```python
from build123d import *

# Parameters (mm, degrees)
SKETCH1_W           = 11.8
SKETCH1_H           = 11.8
BOSS_EXTRUDE1_DEPTH = 10
SKETCH2_R           = 10
BOSS_EXTRUDE2_DEPTH = 3
SKETCH3_R           = 4
BOSS_EXTRUDE3_DEPTH = 15
FILLET1_R           = 0.5
FILLET2_R           = 1.5
CUT_EXTRUDE1_REACH  = 44.389
SKETCH6_R           = 1.1


with BuildPart() as part:
    # Sketch1 → Boss-Extrude1 (new body)
    with BuildSketch(Plane(origin=(0, 0, 0), x_dir=(1, 0, 0), z_dir=(0, 1, 0))):
        Rectangle(SKETCH1_W, SKETCH1_H)
    extrude(amount=BOSS_EXTRUDE1_DEPTH)

    # Sketch2 → Boss-Extrude2 (add)
    with BuildSketch(Plane(origin=(0, 10, 0), x_dir=(1, 0, 0), z_dir=(0, 1, 0))):
        with Locations(Location((0, 0, 0), (0, 0, 270))):
            Circle(SKETCH2_R)
    extrude(amount=BOSS_EXTRUDE2_DEPTH)

    # Sketch3 → Boss-Extrude3 (add)
    with BuildSketch(Plane(origin=(0, 13, 0), x_dir=(1, 0, 0), z_dir=(0, 1, 0))):
        with Locations(Location((0, 0, 0), (0, 0, 270))):
            Circle(SKETCH3_R)
    extrude(amount=BOSS_EXTRUDE3_DEPTH)

    # Sketch4 → Revolve1 (revolve)
    with BuildSketch(Plane.XY):
        with BuildLine():
            Line((0, 38), (0, 22))
            ThreePointArc((0, 22), (8, 30), (0, 38))
        make_face()
    revolve(axis=Axis((0, 0, 0), (0, 1, 0)))

    # Fillet1
    fillet1_edges = [part.edges().sort_by_distance(p)[0] for p in [
        (-5.9, 10, 0),
        (0, 10, 5.9),
        (5.9, 10, 0),
        (0, 10, -5.9),
    ]]
    fillet(fillet1_edges, radius=FILLET1_R)

    # Fillet2
    fillet2_edges = [part.edges().sort_by_distance(p)[0] for p in [
        (0, 13, -4),
    ]]
    fillet(fillet2_edges, radius=FILLET2_R)

    # Sketch6 → Cut-Extrude1 (cut, up to next)
    with BuildSketch(Plane(origin=(5.9, 0, 0), x_dir=(0, 0, -1), z_dir=(1, 0, 0)), mode=Mode.PRIVATE) as cut_extrude1_sk1:
        with Locations((-2.84, 5.28)):
            Circle(SKETCH6_R)
    cut_extrude1_tool1 = extrude(cut_extrude1_sk1.sketch, amount=-CUT_EXTRUDE1_REACH, mode=Mode.PRIVATE) & part.part
    # Sketch6 → Cut-Extrude1 (cut, up to next)
    with BuildSketch(Plane(origin=(5.9, 0, 0), x_dir=(0, 0, -1), z_dir=(1, 0, 0)), mode=Mode.PRIVATE) as cut_extrude1_sk2:
        with Locations((4.16, 5.28)):
            Circle(SKETCH6_R)
    cut_extrude1_tool2 = extrude(cut_extrude1_sk2.sketch, amount=-CUT_EXTRUDE1_REACH, mode=Mode.PRIVATE) & part.part
    add(cut_extrude1_tool1.solids().sort_by_distance((5.9, 5.28, 2.84))[0], mode=Mode.SUBTRACT)
    add(cut_extrude1_tool2.solids().sort_by_distance((5.9, 5.28, -4.16))[0], mode=Mode.SUBTRACT)


solid = part.part
```
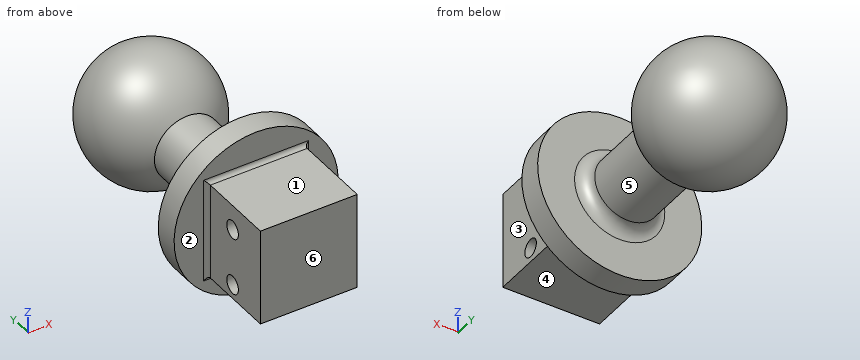
Work out the finished part from the listing and answer in its coordinate system (mm). Face numbers are marked on the shaded views. A direction names the side the tool comes from. Round coordinates to 2 decimals unless told otherwise and drop trailing zeros. Loops run counter-clockwise (first coordinate to the right, second up) from the corner with the lowest first, then second, coordinate; pieces in that order, holes last. Notation, with made-up numbers: (-36, 70) -> (20, 70) arc R20 ccw to (20, 100) -> close; hole circle Ø6 at (-35, 67). An arc over 180 degrees is marked (long way). Write each question's results on one line, items separated by ' | '. Start each with the question number.
1. A tool of negligible diameter and unlimited length cuts with its end or side. For the marked faces 1, 2 and 3, from which of +Z, -Z, +X, -X, +Y, -Y can it reach the whole face along a straight path? Write none if from no direction.
2. For a pull along Y with two mould halves and no side action, classify the marked faces 4, 5 and 6 as +Y half, -Y half, draft (parallel to the pull), parting line (faces both ways), or undercut.
3. Section B-B (x = 0) is taken. Determine the outline of the cut face in (y, z), plus the area to 3 significant figures.
4. Find the intervals of material crossed by probe 1 along Y at (x, z) = (-5.75, 3.75); probe 2 along Y at (x, z) = (3.25, -4.16); probe 3 along Z at (x, y) = (-2.75, 5), in increasing order. Write a range as from..to.
5. Section D-D (x = 4.5) is taken. State how many separate pieces and enclosed holes the cut face has, plus the area to 3 significant figures.
6. Section A-A (y = 5.28) is taken. Determine the outline of the cut face in (x, z), plus the area to 3 significant figures.
7. Given pin 1 Ø7.5 at (x, y) = (-1.5, 5) entering from +Z; pin 2 Ø1 at (x, y) = (1.5, 8) entering from -Z; pin 3 Ø3 at (y, z) = (3.5, 2) entering from +X, each flat-ended and moving along its own axis, determine where each tip first touches the part or whether it passes through.
8. Section C-C (z = 0) is taken. Determine the outline of the cut face in (x, y).
Evaluation:
1) face 1: +Z, +X, -X, -Y | face 2: -Y | face 3: +Z, -Z, +X, -Y
2) face 4: draft | face 5: undercut | face 6: -Y half
3) outline: (0, -5.9) -> (9.5, -5.9) arc R0.5 cw to (10, -6.4) -> (10, -10) -> (13, -10) -> (13, -5.5) arc R1.5 cw to (14.5, -4) -> (23.07, -4) arc R8 ccw (long way) to (23.07, 4) -> (14.5, 4) arc R1.5 cw to (13, 5.5) -> (13, 10) -> (10, 10) -> (10, 6.4) arc R0.5 cw to (9.5, 5.9) -> (0, 5.9) -> close; hole circle Ø2.2 at (5.28, -4.16); hole circle Ø2.2 at (5.28, 2.84) | area: 447 mm2
4) probe 1: y = 0..4.66, 5.9..13, 25.89..34.11 | probe 2: y = 0..4.18, 6.38..13.02, 23.99..36.01 | probe 3: z = -5.9..-5.22, -3.1..1.78, 3.9..5.9
5) separate pieces: 2 | enclosed holes: 2 | area: 303 mm2
6) outline: (-5.9, -5.9) -> (5.9, -5.9) -> (5.9, -5.26) -> (-5.9, -5.26) -> close; (-5.9, -3.06) -> (5.9, -3.06) -> (5.9, 1.74) -> (-5.9, 1.74) -> close; (-5.9, 3.94) -> (5.9, 3.94) -> (5.9, 5.9) -> (-5.9, 5.9) -> close | area: 87.3 mm2
7) pin 1: stops at z = 5.9 | pin 2: stops at z = -5.9 | pin 3: stops at x = 5.9
8) outline: (-10, 10) -> (-6.4, 10) arc R0.5 cw to (-5.9, 9.5) -> (-5.9, 0) -> (5.9, 0) -> (5.9, 9.5) arc R0.5 cw to (6.4, 10) -> (10, 10) -> (10, 13) -> (5.5, 13) arc R1.5 cw to (4, 14.5) -> (4, 23.07) arc R8 ccw (long way) to (-4, 23.07) -> (-4, 14.5) arc R1.5 cw to (-5.5, 13) -> (-10, 13) -> close
